from build123d import *

# Parameters (mm, degrees)
BOSS_EXTRUDE1_DEPTH              = 25.4
SKETCH4_W                        = 80
SKETCH4_H                        = 50
CUT_EXTRUDE1_DEPTH               = 15
FILLET1_R                        = 10
F_12_0MM_DOWEL_HOLE1_D           = 12
F_12_0MM_DOWEL_HOLE1_CSINK_D     = 12.05
F_12_0MM_DOWEL_HOLE1_CSINK_ANGLE = 100


with BuildPart() as part:
    # Sketch1 → Boss-Extrude1 (new body)
    with BuildSketch(Plane(origin=(0, 0, 0), x_dir=(1, 0, 0), z_dir=(0, 1, 0))):
        Polygon((-150, 65), (-140, 75), (140, 75), (150, 65), (150, -65), (140, -75), (-140, -75), (-150, -65), align=None)
    extrude(amount=BOSS_EXTRUDE1_DEPTH)

    # Sketch4 → Cut-Extrude1 (cut)
    with BuildSketch(Plane(origin=(0, 25.4, 0), x_dir=(1, 0, 0), z_dir=(0, 1, 0))):
        Rectangle(SKETCH4_W, SKETCH4_H)
    extrude(amount=-CUT_EXTRUDE1_DEPTH, mode=Mode.SUBTRACT)

    # Fillet1
    fillet1_edges = [part.edges().sort_by_distance(p)[0] for p in [
        (40, 17.9, -25),
        (40, 17.9, 25),
        (-40, 17.9, 25),
        (-40, 17.9, -25),
    ]]
    fillet(fillet1_edges, radius=FILLET1_R)

    # Ø12.0mm Dowel Hole1 (through all)
    with Locations(Plane(origin=(0, 25.4, 0), x_dir=(1, 0, 0), z_dir=(0, 1, 0))):
        with Locations((-125, 50), (125, 50), (125, -50), (-125, -50)):
            CounterSinkHole(F_12_0MM_DOWEL_HOLE1_D / 2, F_12_0MM_DOWEL_HOLE1_CSINK_D / 2, counter_sink_angle=F_12_0MM_DOWEL_HOLE1_CSINK_ANGLE)


solid = part.part
Can you work these out from the model? Positions are in its coordinate system, mm. A direction names the side the tool comes from. Give positions to 0.01 mm unless a question says otherwise; leave off trailing zeros. Loops run counter-clockwise (first coordinate to the right, second up) from the corner with the lowest first, then second, coordinate; pieces in that order, holes last. Notation, with made-up numbers: M 40.25,-24.75 L 73.25,-24.75 A20 ccw 73.25,-13.75 Z; hole C 52.5,45 d10. An arc over 180 degrees is marked long. One line per item, written item: value.
1) Imagine slicing it at A-A on z = 50. Write out the boundary of the cut face in (x, y) (3 decimals), and give its area (3 significant figures).
Geometry check:
outline: M -150,0 L -131,0 L -131,25.379 L -131.025,25.4 L -150,25.4 Z; M -119,0 L 119,0 L 119,25.379 L 118.975,25.4 L -118.975,25.4 L -119,25.379 Z; M 131,0 L 150,0 L 150,25.4 L 131.025,25.4 L 131,25.379 Z
area: 7,010 mm²
2) Thinking about a two-plate mould opening in X: for faces 3 (the face through (-37.15, 17.79, 21.99)), 4 (the face through (145, 13, 70)), 5 (the face through (-37.15, 17.79, -21.99)), 6 (the face through (2, 13, 75)), which applies, +X half, -X half, draft (parallel to the pull), parting line (faces both ways), or undercut?
Geometry check:
face 3: undercut
face 4: +X half
face 5: undercut
face 6: draft
3) Imagine slicing it at C-C on x = 125. Write out the boundary of the cut face in (y, z) (3 decimals).
Geometry check:
outline: M 0,-75 L 25.4,-75 L 25.4,-56.025 L 25.379,-56 L 0,-56 Z; M 0,-44 L 25.379,-44 L 25.4,-43.975 L 25.4,43.975 L 25.379,44 L 0,44 Z; M 0,56 L 25.379,56 L 25.4,56.025 L 25.4,75 L 0,75 Z
4) On a 3-axis mill with a long thin cutter (end or side, diameter ignored), from which of +Z, -Z, +X, -X, +Y, -Y can I reach the whole of each face in a straight line? I mean faces 1 (the face through (40, 18, 0)), 2 (the face through (-119, 13, -50)). Say none if no direction works.
Geometry check:
face 1: +Y
face 2: +Y, -Y
5) Imagine slicing it at B-B on y = 20.25. Write out the boundary of the cut face in (x, z), and give its area (3 significant figures).
Geometry check:
outline: M -150,-65 L -140,-75 L 140,-75 L 150,-65 L 150,65 L 140,75 L -140,75 L -150,65 Z; hole C -125,-50 d12; hole C -125,50 d12; hole M -40,-15 A10 ccw -30,-25 L 30,-25 A10 ccw 40,-15 L 40,15 A10 ccw 30,25 L -30,25 A10 ccw -40,15 Z; hole C 125,-50 d12; hole C 125,50 d12
area: 40,400 mm²
6) Please list where these lines run through material, in increasing order: line 1 (Z direction, x = 125, y = 18.75); line 2 (X direction, y = 6.5, z = 50); line 3 (X direction, y = 17.25, z = -1).
Geometry check:
line 1: z = -75 to -56, -44 to 44, 56 to 75
line 2: x = -150 to -131, -119 to 119, 131 to 150
line 3: x = -150 to -40, 40 to 150
7) Imagine slicing it at D-D on z = 18.5. Write out the boundary of the cut face in (x, y), and give its area (3 significant figures).
Geometry check:
outline: M -150,0 L 150,0 L 150,25.4 L 39.37,25.4 L 39.37,10.4 L -39.37,10.4 L -39.37,25.4 L -150,25.4 Z
area: 6,440 mm²
